Can you work these out from the drawing? Everything is in mm from the part's minimum corner. A direction names the side the tool comes from. Give positions to 0.01 mm unless a question says otherwise; leave off trailing zeros. Write each loop counter-clockwise with the first axis right and the second up, starting at its lowest first coordinate (ties: lowest second). Pieces come first, ordered by that corner, then holes. Notation, with made-up numbers: M 67,56 L 98,56 A19 cw 98,85 Z; hole C 46,46.25 d10. An arc over 180 degrees is marked long. One line per item, written item: value.
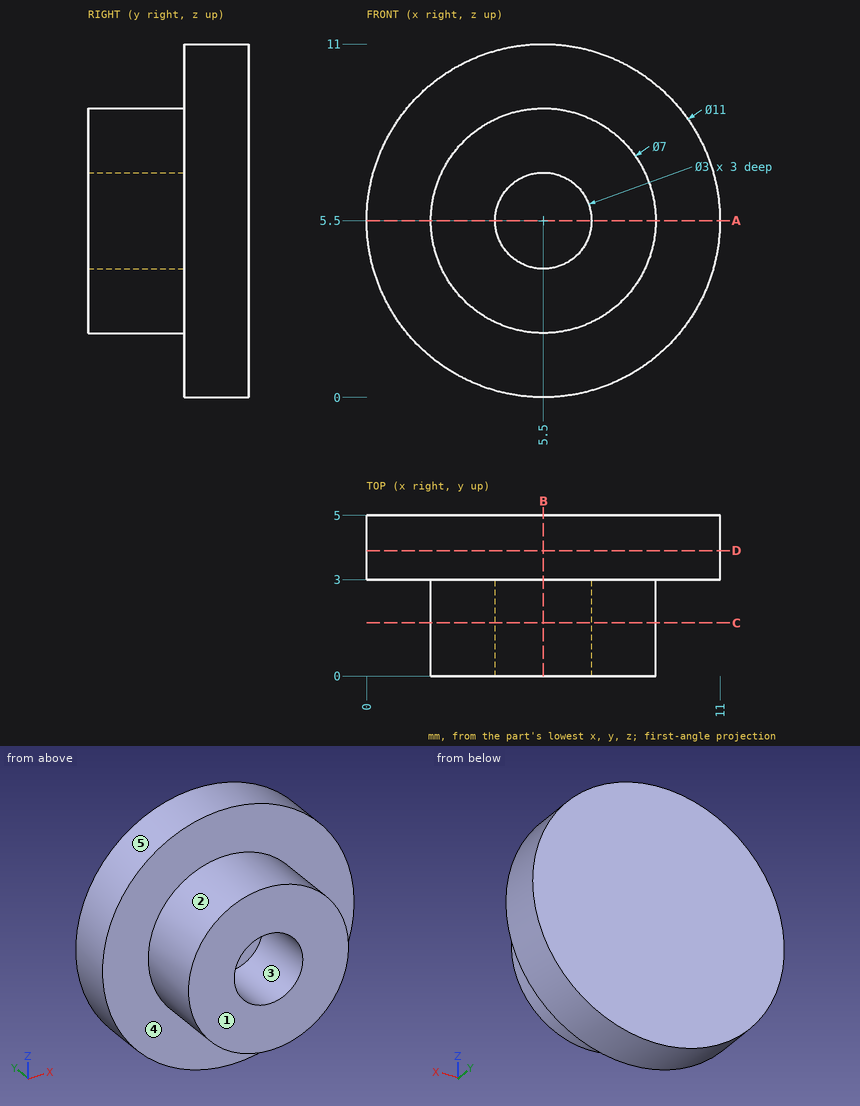
1) If we section it at C-C, the plane y = 1.65: Write out the boundary of the cut face in (x, z), then the cut area to 3 significant figures.
Outcome:
outline: C 5.5,5.5 d7; hole C 5.5,5.5 d3
area: 31.4 mm^2
2) If we section it at B-B, the plane x = 5.5: Write out the boundary of the cut face in (y, z), then the cut area to 3 significant figures.
Outcome:
outline: M 0,2 L 3,2 L 3,0 L 5,0 L 5,11 L 3,11 L 3,9 L 0,9 L 0,7 L 3,7 L 3,4 L 0,4 Z
area: 34.0 mm^2
3) Please list where these lines run through material, in increasing order: L1, parallel to Z at x = 5.5, y = 1.2; L2, parallel to Y at x = 8, z = 8.5. Write a range as from..to.
Outcome:
L1: z = 2..4, 7..9
L2: y = 3..5
4) On a 3-axis mill with a long thin cutter (end or side, diameter ignored), from which of +Z, -Z, +X, -X, +Y, -Y can I reach the whole of each face in a straight line? I mean the marked faces 4 and 5. Say none if no direction works.
Outcome:
face 4: -Y
face 5: +Y, -Y
5) I'm going to push flat-ended pins straight in: pin 1 (3 mm diameter, centred on x = 7, z = 4, fed in from -Y); pin 2 (0.9 mm diameter, centred on x = 5, z = 5.5, fed in from -Y). Where does each tip first touch, or does it pass through?
Outcome:
pin 1: stops at y = 0
pin 2: stops at y = 3
6) If we section it at A-A, the plane z = 5.5: Write out the boundary of the cut face in (x, y), then the cut area to 3 significant figures.
Outcome:
outline: M 0,3 L 2,3 L 2,0 L 4,0 L 4,3 L 7,3 L 7,0 L 9,0 L 9,3 L 11,3 L 11,5 L 0,5 Z
area: 34.0 mm^2
7) If we section it at D-D, the plane y = 3.9: Write out the boundary of the cut face in (x, z).
Outcome:
outline: C 5.5,5.5 d11
8) We'd pull the mould along X, two halves only. Please class the marked faces 1, 2 and 3: pulls with the +X half, pulls with the -X half, needs draft (parallel to the pull), parting line crosses it, or undercut.
Outcome:
face 1: needs draft
face 2: parting line crosses it
face 3: undercut
